Here's how the part is built. I have some questions about the finished solid (model axes, mm). A direction names the side the tool comes from. Round coordinates to 2 decimals unless told otherwise and drop trailing zeros. Write each loop counter-clockwise with the first axis right and the second up, starting at its lowest first coordinate (ties: lowest second). Pieces come first, ordered by that corner, then holes. Notation, with made-up numbers: M 66,79 L 109,79 A36 ccw 109,117 Z; hole C 68,-15 d8. An arc over 180 degrees is marked long. Write item = value, one per line. Start each with the question number.
(1) I want a section at B-B (y = 1.5). List the corners of the cut face in (x, z) for me, and give its area (3 significant figures).
(2) If we mould it in two halves opening along X, with no side actions, what happens to faces 1 (the cylindrical face through (-15.8, 1.9, 84.6)), 2 (the flat face through (-20.724, 1, 55)), 3 (the flat face through (-16, 0, 55))? For each: released by +X, released by -X, zero draft, split by the parting line, or undercut.
(3) I want a section at C-C (z = 81). List the corners of the cut face in (x, y) for me.
(4) I want a section at A-A (z = 25.4). List the corners of the cut face in (x, y) for me, and give its area (3 significant figures).
(5) I want a section at D-D (y = 8.5). List the corners of the cut face in (x, z) for me, and give its area (3 significant figures).
(6) Will these pins go through, and if not, where does the flat tip stop? pin 1 Ø2 at (y, z) = (2.5, 78) entering from +X; pin 2 Ø2 at (x, z) = (-15.5, 60) entering from +Y; pin 3 Ø3 at (y, z) = (7, 14.5) entering from +X.
(7) On a 3-axis mill with a long thin cutter (end or side, diameter ignored), from which of +Z, -Z, +X, -X, +Y, -Y can I reach the whole of each face in a straight line? I mean faces 4 (the flat face through (12, 0, 55)), 5 (the flat face through (-16, 3.81, 55)). Say none if no direction works.
(8) I need wall thicknesses on line 1 along X through (y, z) = (2, 25.4); line 2 along X through (y, z) = (0.8, 25.4); line 3 along Y through (x, z) = (-12.5, 98.5). Which ranges of each line are inside material? Lowest first, please.
```python
from build123d import *

# Parameters (mm, degrees)
BOSS_EXTRUDE1_DEPTH = 112
SKETCH3_R           = 2
CUT_EXTRUDE2_DEPTH  = 115.271427971
FILLET1_R           = 1.27


with BuildPart() as part:
    # Sketch1 → Boss-Extrude1 (new body)
    with BuildSketch(Plane.XY):
        with BuildLine():
            ThreePointArc((-12.429155241, 3.81), (-12.856496765, 1.926263465), (-13, 0))
            Line((-13, 0), (-11, 0))
            ThreePointArc((-11, 0), (0, 11), (11, 0))
            Line((11, 0), (13, 0))
            ThreePointArc((13, 0), (9.192388155, 9.192388155), (0, 13))
            ThreePointArc((0, 13), (-7.728842087, 10.452990003), (-12.429155241, 3.81))
        make_face()
        with BuildLine():
            Line((-20.724457785, 0), (-13, 0))
            ThreePointArc((-13, 0), (-12.856496765, 1.926263465), (-12.429155241, 3.81))
            Line((-12.429155241, 3.81), (-20.724457785, 3.81))
            Line((-20.724457785, 3.81), (-20.724457785, 0))
        make_face()
    extrude(amount=BOSS_EXTRUDE1_DEPTH)

    # Sketch3 → Cut-Extrude2 (cut, through all)
    with BuildSketch(Plane(origin=(0, 3.81, 0), x_dir=(1, 0, 0), z_dir=(0, 1, 0))):
        with Locations(Location((-15.862228893, -25.4, 0), (0, 0, 270))):
            Circle(SKETCH3_R)
        with Locations(Location((-15.862228893, -86.6, 0), (0, 0, 270))):
            Circle(SKETCH3_R)
    extrude(amount=-CUT_EXTRUDE2_DEPTH, mode=Mode.SUBTRACT)

    # Fillet1
    fillet1_edges = [part.edges().sort_by_distance(p)[0] for p in [
        (-20.724457785, 3.81, 56),
    ]]
    fillet(fillet1_edges, radius=FILLET1_R)


solid = part.part
```
Returned:
q1.outline = M -20.72,0 L -10.9,0 L -10.9,112 L -20.72,112 Z; M 10.9,0 L 12.91,0 L 12.91,112 L 10.9,112 Z; hole C -15.86,25.4 d4; hole C -15.86,86.6 d4
q1.area = 1,300 mm²
q2.face_1 = undercut
q2.face_2 = released by -X
q2.face_3 = zero draft
q3.outline = M -20.72,0 L -11,0 A11 cw 11,0 L 13,0 A13 ccw -12.43,3.81 L -19.45,3.81 A1.27 ccw -20.72,2.54 Z
q4.outline = M -20.72,0 L -17.86,0 L -17.86,3.81 L -19.45,3.81 A1.27 ccw -20.72,2.54 Z; M -13.86,0 L -11,0 A11 cw 11,0 L 13,0 A13 ccw -12.43,3.81 L -13.86,3.81 Z
q4.area = 90.0 mm²
q5.outline = M -9.84,0 L -6.98,0 L -6.98,112 L -9.84,112 Z; M 6.98,0 L 9.84,0 L 9.84,112 L 6.98,112 Z
q5.area = 639 mm²
q6.pin_1 = 12.91
q6.pin_2 = 3.81
q6.pin_3 = 11.78
q7.face_4 = +Z, -Z, +X, -X, -Y
q7.face_5 = +Z, -Z, -X, +Y
q8.line_1 = -20.72 to -17.86, -13.86 to -10.82, 10.82 to 12.85
q8.line_2 = -20.72 to -17.86, -13.86 to -10.97, 10.97 to 12.98
q8.line_3 = 0 to 3.81
